Geometry check sheet. Reference: drawing and pictorial views, mm from the part's lowest x, y, z. Give positions to 0.01 mm unless a question says otherwise; leave off trailing zeros. Loops run counter-clockwise (first coordinate to the right, second up) from the corner with the lowest first, then second, coordinate; pieces in that order, holes last. Notation, with made-up numbers: (-6.75, 51) -> (0.25, 51) arc R19 ccw to (0.25, 78) -> close; hole circle Ø6 at (-14.75, 9.25). An arc over 180 degrees is marked (long way). Answer in a Markdown table with one row per item. Add a question column.
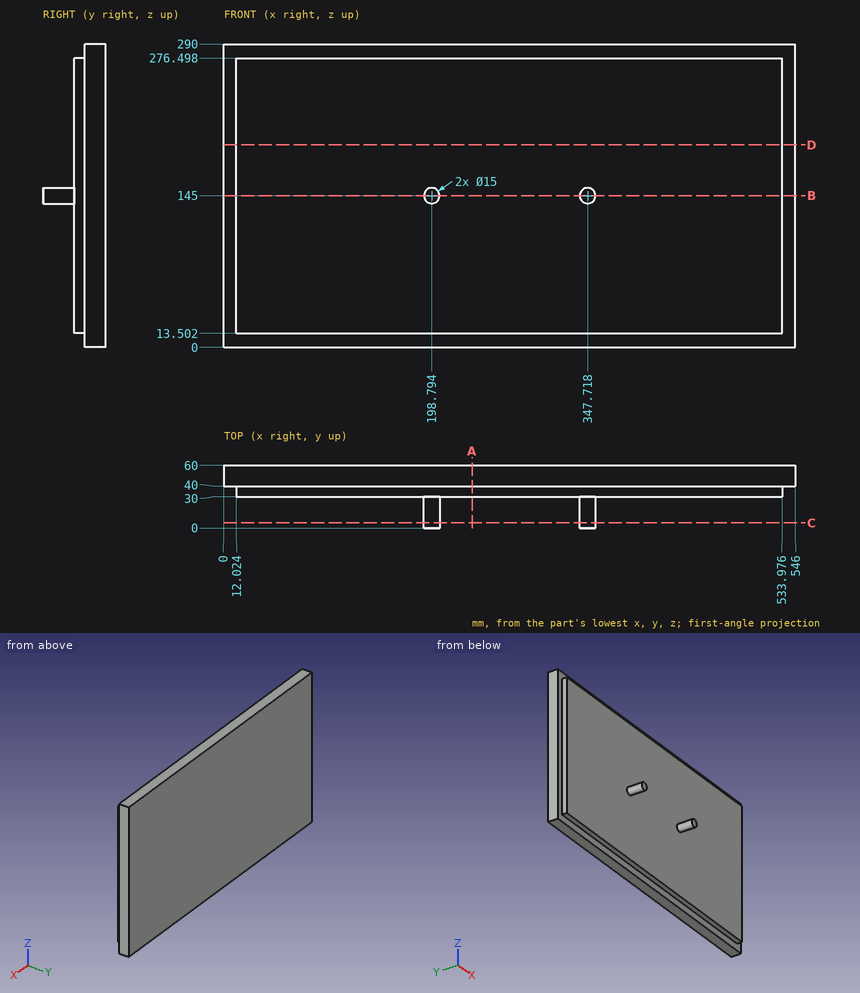
1. Sectioned sample at C-C (y = 5). Enter the section's corners in (x, z) (1 decimal).
2. Sectioned sample at B-B (z = 145). Enter the section's corners in (x, y) (1 decimal).
3. Sectioned sample at A-A (x = 237.5). Enter the section's corners in (y, z).
4. Gauge pin test, flat ends, axial feed: pin 1 Ø3 at (y, z) = (32.5, 84) entering from +X; pin 2 Ø11 at (x, y) = (195, 37.5) entering from -Z; pin 3 Ø5 at (x, y) = (254.5, 33) entering from +Z; pin 4 Ø3 at (y, z) = (37, 173) entering from -X. Record the tip position at first contact, or that the pin passes through.
5. Material ranges on L1, parallel to X at y = 31, z = 36 (1 decimal); L2, parallel to Z at x = 57.5, y = 36; L3, parallel to Y at x = 209.5, z = 71, recorded low to high. Write a range as from..to.
6. Sectioned sample at D-D (z = 193.5). Enter the section's corners in (x, y) (1 decimal).
Response:
| question | item | result |
|---|---|---|
| 1 | outline | circle Ø15 at (198.8, 145); circle Ø15 at (347.7, 145) |
| 2 | outline | (0, 40) -> (12, 40) -> (12, 30) -> (191.3, 30) -> (191.3, 0) -> (206.3, 0) -> (206.3, 30) -> (340.2, 30) -> (340.2, 0) -> (355.2, 0) -> (355.2, 30) -> (534, 30) -> (534, 40) -> (546, 40) -> (546, 60) -> (0, 60) -> close |
| 3 | outline | (30, 13.5) -> (40, 13.5) -> (40, 0) -> (60, 0) -> (60, 290) -> (40, 290) -> (40, 276.5) -> (30, 276.5) -> close |
| 4 | pin 1 | stops at x = 533.98 |
| 4 | pin 2 | stops at z = 0 |
| 4 | pin 3 | stops at z = 276.5 |
| 4 | pin 4 | stops at x = 12.02 |
| 5 | L1 | x = 12..534 |
| 5 | L2 | z = 13.5..276.5 |
| 5 | L3 | y = 30..60 |
| 6 | outline | (0, 40) -> (12, 40) -> (12, 30) -> (534, 30) -> (534, 40) -> (546, 40) -> (546, 60) -> (0, 60) -> close |
